Geometry check sheet. Reference: the model listing, model coordinates, mm. A direction names the side the tool comes from. Round coordinates to 2 decimals unless told otherwise and drop trailing zeros. Write each loop counter-clockwise with the first axis right and the second up, starting at its lowest first coordinate (ties: lowest second). Pieces come first, ordered by that corner, then holes. Notation, with made-up numbers: M 38.25,11 L 83.25,11 A17 ccw 83.25,19 Z; hole C 79.25,66 d9. An arc over 180 degrees is marked long. Use a Markdown table: item, result.
```python
from build123d import *

# Parameters (mm, degrees)
SKETCH_W        = 49.4
SKETCH_H        = 148
SKETCH_R        = 1.75
SKETCH_R_2      = 23.5
SKETCH_R_3      = 13
PAD_DEPTH       = 3
CHAMFER_SIZE    = 2.6
SKETCH001_R     = 3.1
POCKET_DEPTH    = 2.1
SKETCH002_R     = 15.51
PAD001_DEPTH    = 15
SKETCH003_R     = 13
POCKET001_DEPTH = 13
SKETCH004_R     = 4
POCKET002_DEPTH = 15.001


with BuildPart() as part:
    # Sketch → Pad (new body)
    with BuildSketch(Plane.XY):
        with Locations((24.7, 74)):
            Rectangle(SKETCH_W, SKETCH_H)
        with Locations((24.7, 126.745966)):
            Circle(SKETCH_R, mode=Mode.SUBTRACT)
        with Locations((24.7, 65.745966)):
            Circle(SKETCH_R, mode=Mode.SUBTRACT)
        with Locations((24.7, 96.245966)):
            Circle(SKETCH_R_2, mode=Mode.SUBTRACT)
        with Locations((4.7, 143.3)):
            Circle(SKETCH_R, mode=Mode.SUBTRACT)
        with Locations((44.7, 143.3)):
            Circle(SKETCH_R, mode=Mode.SUBTRACT)
        with Locations((4.7, 4.7)):
            Circle(SKETCH_R, mode=Mode.SUBTRACT)
        with Locations((44.7, 4.7)):
            Circle(SKETCH_R, mode=Mode.SUBTRACT)
        with Locations((24.7, 26)):
            Circle(SKETCH_R_3, mode=Mode.SUBTRACT)
    extrude(amount=PAD_DEPTH)

    # Chamfer
    chamfer_edges = [part.edges().sort_by_distance(p)[0] for p in [
        (2.95, 4.7, 0),
        (42.95, 4.7, 0),
        (22.95, 65.745966, 0),
        (22.95, 126.745966, 0),
        (2.95, 143.3, 0),
        (42.95, 143.3, 0),
    ]]
    chamfer(chamfer_edges, length=CHAMFER_SIZE)

    # Sketch001 → Pocket (cut)
    with BuildSketch(Plane.XY):
        with Locations((24.7, 142)):
            Circle(SKETCH001_R)
        with Locations((24.7, 6)):
            Circle(SKETCH001_R)
        with Locations((43.4, 26)):
            Circle(SKETCH001_R)
        with Locations((6, 26)):
            Circle(SKETCH001_R)
        with Locations((6, 58)):
            Circle(SKETCH001_R)
        with Locations((43.159603, 58)):
            Circle(SKETCH001_R)
    extrude(amount=POCKET_DEPTH, mode=Mode.SUBTRACT)

    # Sketch002 → Pad001 (join)
    with BuildSketch(Plane.XY):
        with Locations((24.7, 26)):
            Circle(SKETCH002_R)
    extrude(amount=PAD001_DEPTH)

    # Sketch003 → Pocket001 (cut)
    with BuildSketch(Plane.XY):
        with Locations((24.7, 26)):
            Circle(SKETCH003_R)
    extrude(amount=POCKET001_DEPTH, mode=Mode.SUBTRACT)

    # Sketch004 → Pocket002 (cut, through all)
    with BuildSketch(Plane.XY):
        with Locations((24.7, 26)):
            Circle(SKETCH004_R)
    extrude(amount=POCKET002_DEPTH, mode=Mode.SUBTRACT)


solid = part.part
```
Item 1: Mould release check, pull along Y, two halves, no side actions. Record for faces 4 (the face through (24, 148, 1)), 5 (the face through (24, 59, 0)), 6 (the face through (42.95, 4.78, 2.8)): +Y half, -Y half, draft (parallel to the pull), parting line (faces both ways), or undercut.
Outcome:
| item | result |
|---|---|
| face 4 | +Y half |
| face 5 | draft |
| face 6 | undercut |
Item 2: Cross-section at D-D, the plane x = 24.7. Count the separate pieces of the cut face and the enclosed holes in it, and give its area (3 significant figures).
Outcome:
| item | result |
|---|---|
| separate pieces | 5 |
| enclosed holes | 0 |
| area | 261 mm2 |
Item 3: Go/stop test with flat-tipped pins: pin 1 (4 mm diameter, centred on x = 27, z = 4.5, fed in from -Y); pin 2 (1 mm diameter, centred on x = 14.5, z = 9, fed in from +Y); pin 3 (5.5 mm diameter, centred on x = 6, y = 26, fed in from +Z); pin 4 (2 mm diameter, centred on x = 34, z = 9, fed in from -Y). Record where each tip stops, or that it passes through.
Outcome:
| item | result |
|---|---|
| pin 1 | stops at y = 0 |
| pin 2 | stops at y = 38.1 |
| pin 3 | stops at z = 3 |
| pin 4 | stops at y = 12.9 |
Item 4: Cross-section at C-C, the plane z = 9. Record the cut outline in (x, y), and give its area (3 significant figures).
Outcome:
| item | result |
|---|---|
| outline | C 24.7,26 d31.02; hole C 24.7,26 d26 |
| area | 225 mm2 |
Item 5: Material ranges on line 1 along Y through (x, z) = (24, 5); line 2 along Y through (x, z) = (24.7, 13.6); line 3 along Y through (x, z) = (44.7, 2.75), recorded low to high. Write a range as from..to.
Outcome:
| item | result |
|---|---|
| line 1 | y = 10.51..13.02, 38.98..41.49 |
| line 2 | y = 10.49..22, 30..41.51 |
| line 3 | y = 0..2.95, 6.45..83.91, 108.58..141.55, 145.05..148 |
Item 6: Cross-section at B-B, the plane y = 58. Record the cut outline in (x, z), and give its area (3 significant figures).
Outcome:
| item | result |
|---|---|
| outline | M 0,0 L 2.9,0 L 2.9,2.1 L 9.1,2.1 L 9.1,0 L 40.06,0 L 40.06,2.1 L 46.26,2.1 L 46.26,0 L 49.4,0 L 49.4,3 L 0,3 Z |
| area | 122 mm2 |
Item 7: Access from +Z, -Z, +X, -X, +Y, -Y to the whole of each face (thin tool, end or side, straight path). Record for faces 1 (the face through (24.296, 145.074, 1.035)), 2 (the face through (31.86, 12.24, 8.92)), 3 (the face through (0, 73, 1)).
Outcome:
| item | result |
|---|---|
| face 1 | -Z |
| face 2 | +Z |
| face 3 | +Z, -Z, -X, +Y, -Y |
Item 8: Cross-section at A-A, the plane x = 4.7. Record the cut outline in (y, z).
Outcome:
| item | result |
|---|---|
| outline | M 0,0 L 0.35,0 L 2.95,2.6 L 2.95,3 L 0,3 Z; M 6.45,2.6 L 9.05,0 L 23.19,0 L 23.19,2.1 L 28.81,2.1 L 28.81,0 L 55.19,0 L 55.19,2.1 L 60.81,2.1 L 60.81,0 L 83.91,0 L 83.91,3 L 6.45,3 Z; M 108.58,0 L 138.95,0 L 141.55,2.6 L 141.55,3 L 108.58,3 Z; M 145.05,2.6 L 147.65,0 L 148,0 L 148,3 L 145.05,3 Z |
